```python
from build123d import *

# Parameters (mm, degrees)
F0_W      = 4.572
F0_H      = 2.032
F1_DEPTH  = 1.6
F3_DEPTH  = 12.192
F4_DEPTH  = 3.175
F5_DEPTH  = 0.508
F6_DEPTH  = 0.508
F7_DEPTH  = 0.508
F8_DEPTH  = 0.508
F9_DEPTH  = 0.127
F11_DEPTH = 1.5875
F13_DEPTH = 12.319
F14_DEPTH = 3.175


# Not quite as in the source:
# - a feature of the source that left no trace in its solid (it failed there, or was rolled back) is left out
# - a pattern or mirror of a feature is missing from the dataset's text; its kind, count and spacing are read off the source's solid


with BuildPart() as f1:
    # F0 (on Top) → F1 (new body)
    with BuildSketch(Plane.XY):
        Polygon((0, -2.032), (0, 0), (4.572, 0), (4.572, 3.556), (-1.6, 3.556), (-1.6, -1.016), (-1.6, -5.588), (4.572, -5.588), (4.572, -2.032), align=None)
        Polygon((33.858, 3.556), (27.686, 3.556), (27.686, 0), (32.258, 0), (32.258, -2.032), (27.686, -2.032), (27.686, -5.588), (33.858, -5.588), (33.858, -1.016), align=None)
        Polygon((4.572, 3.556), (4.572, 0), (4.572, -2.032), (4.572, -5.588), (27.686, -5.588), (27.686, -2.032), (27.686, 0), (27.686, 3.556), align=None)
        with Locations((2.286, -1.016)):
            Rectangle(F0_W, F0_H)
        with Locations((29.972, -1.016)):
            Rectangle(F0_W, F0_H)
    extrude(amount=F1_DEPTH)

    # F2 (on face) → F3 (join)
    with BuildSketch(Plane.XY.offset(1.6)):
        Polygon((0, -2.032), (0, 0), (4.572, 0), (4.572, 3.556), (-1.6, 3.556), (-1.6, -1.016), (-1.6, -5.588), (4.572, -5.588), (4.572, -2.032), align=None)
        Polygon((33.858, 3.556), (27.686, 3.556), (27.686, 0), (32.258, 0), (32.258, -2.032), (27.686, -2.032), (27.686, -5.588), (33.858, -5.588), (33.858, -1.016), align=None)
    extrude(amount=F3_DEPTH)

    # F4 (add): a face of the model
    f4_faces = [f1.faces().sort_by_distance(p)[0] for p in [
        (-1.2195411943, -5.588, 6.896),
    ]]
    extrude(f4_faces, amount=F4_DEPTH)

    # F5 (add): a face of the model
    f5_faces = [f1.faces().sort_by_distance(p)[0] for p in [
        (-1.6, -2.6035, 6.896),
    ]]
    extrude(f5_faces, amount=F5_DEPTH)

    # F6 (cut): a face of the model
    f6_faces = [f1.faces().sort_by_distance(p)[0] for p in [
        (0, -1.016, 7.696),
    ]]
    extrude(f6_faces, amount=-F6_DEPTH, mode=Mode.SUBTRACT)

    # F7 (add): a face of the model
    f7_faces = [f1.faces().sort_by_distance(p)[0] for p in [
        (33.858, -2.6035, 6.896),
    ]]
    extrude(f7_faces, amount=F7_DEPTH)

    # F8 (cut): a face of the model
    f8_faces = [f1.faces().sort_by_distance(p)[0] for p in [
        (32.258, -1.016, 7.696),
    ]]
    extrude(f8_faces, amount=-F8_DEPTH, mode=Mode.SUBTRACT)

    # F9 (cut): faces of the model
    f9_faces = [f1.faces().sort_by_distance(p)[0] for p in [
        (4.572, -5.3975, 7.696),
        (4.572, 1.778, 7.696),
    ]]
    f9 = extrude(f9_faces, amount=-F9_DEPTH, mode=Mode.SUBTRACT)

    # F9_copies: F9 across plane
    add(f9.mirror(Plane(origin=(16.129, 0, 0), x_dir=(0, 0, 1), z_dir=(1, 0, 0))), mode=Mode.SUBTRACT)

    # F11 (add): a face of the model
    f11_faces = [f1.faces().sort_by_distance(p)[0] for p in [
        (16.129, -2.6035, 0),
    ]]
    extrude(f11_faces, amount=F11_DEPTH)

    # F12 (on face) → F13 (join, through all)
    with BuildSketch(Plane.XZ.offset(8.763)):
        Polygon((-2.108, -1.5875), (-2.108, 13.792), (-17.475, -1.5875), align=None)
        Polygon((49.733, -1.5875), (34.366, 13.792), (34.366, -1.5875), align=None)
    extrude(amount=-F13_DEPTH)

    # F14 (add): a face of the model
    f14_faces = [f1.faces().sort_by_distance(p)[0] for p in [
        (16.129, -2.6035, -1.5875),
    ]]
    extrude(f14_faces, amount=F14_DEPTH)


solid = f1.part
```
CAD build for the part. Positions are in the model's coordinates, mm. A direction names the side the tool comes from. Give positions to 0.01 mm unless a question says otherwise; leave off trailing zeros. Write each loop counter-clockwise with the first axis right and the second up, starting at its lowest first coordinate (ties: lowest second). Pieces come first, ordered by that corner, then holes. Notation, with made-up numbers: M 65.25,22 L 120.25,22 A5 ccw 120.25,26 Z; hole C -17,47.5 d4. An arc over 180 degrees is marked long. Return JSON: item names as keys, results as strings. Group by question number.
(1) Band-saw the part on D-D (z = 8.75). Give the cut face in (x, y) (3 decimals).
(2) Band-saw the part on C-C (x = 25.5). Give the cut face in (y, z), and give its area (3 significant figures).
(3) Band-saw the part on A-A (z = 3). Give the cut face in (x, y) (3 decimals), and give its area (3 significant figures).
(4) Mould opens along Y. For faces 1 (the face through (27.813, -5, 8)), 2 (the face through (17, -8.763, 1)), 3 (the face through (30, 0, 8)) say: pulls with the +Y half, pulls with the -Y half, needs draft (parallel to the pull), parting line crosses it, or undercut.
(5) Drill centre lines: L1, parallel to Y at x = 31, z = 2; L2, parallel to Z at x = 19.5, y = -7; L3, parallel to X at y = -2.5, z = 3.5 (3 decimals). Where is each one in solid material? Low to high. Write a range as [from, to].
(6) 3-axis set-ups, long thin cutter, end or side, ignore diameter. For faces 4 (the face through (-9.684, -2.69, 6.21)), 5 (the face through (4.445, 2, 8)), 6 (the face through (30, -2.032, 8)): which of +Z, -Z, +X, -X, +Y, -Y reach the whole face in a straight line?
(7) Band-saw the part on B-B (y = -1). Give the cut face in (x, z) (1 decimal).
(8) Flat gauge pins, fed straight in: pin 1 Ø4 at (y, z) = (2.5, 6) entering from -X; pin 2 Ø3.5 at (y, z) = (-4.5, 5.5) entering from -X; pin 3 Ø1 at (y, z) = (-5.5, 4.5) entering from +X. Where does each tip first touch, or does it go through?
Entries:
{
 "1": {"outline": "M -7.146,-8.763 L 4.445,-8.763 L 4.445,-2.032 L -0.508,-2.032 L -0.508,0 L 4.445,0 L 4.445,3.556 L -7.146,3.556 Z; M 27.813,-8.763 L 39.404,-8.763 L 39.404,3.556 L 27.813,3.556 L 27.813,0 L 32.766,0 L 32.766,-2.032 L 27.813,-2.032 Z"},
 "2": {"outline": "M -8.76,-4.76 L 3.56,-4.76 L 3.56,1.6 L -8.76,1.6 Z", "area": "78.4 mm^2"},
 "3": {"outline": "M -12.891,-8.763 L 4.445,-8.763 L 4.445,-2.032 L -0.508,-2.032 L -0.508,0 L 4.445,0 L 4.445,3.556 L -12.891,3.556 Z; M 27.813,-8.763 L 45.149,-8.763 L 45.149,3.556 L 27.813,3.556 L 27.813,0 L 32.766,0 L 32.766,-2.032 L 27.813,-2.032 Z", "area": "407 mm^2"},
 "4": {"face 1": "needs draft", "face 2": "pulls with the -Y half", "face 3": "undercut"},
 "5": {"L1": "y = [-8.76, -2.03], [0, 3.56]", "L2": "z = [-4.76, 1.6]", "L3": "x = [-12.392, 4.445], [27.813, 44.65]"},
 "6": {"face 4": "+Z, -X, +Y, -Y", "face 5": "+Z, +Y, -Y", "face 6": "+Z"},
 "7": {"outline": "M -17.5,-4.8 L 49.7,-4.8 L 49.7,-1.6 L 34.4,13.8 L 32.8,13.8 L 32.8,1.6 L -0.5,1.6 L -0.5,13.8 L -2.1,13.8 L -17.5,-1.6 Z"},
 "8": {"pin 1": "stops at x = -11.89", "pin 2": "stops at x = -12.14", "pin 3": "stops at x = 44.15"}
}
